Here's the drawing with two shaded views (mm, measured from the low corner). I have some questions. Round coordinates to 2 decimals unless told otherwise and drop trailing zeros. Loops run counter-clockwise (first coordinate to the right, second up) from the corner with the lowest first, then second, coordinate; pieces in that order, holes last.
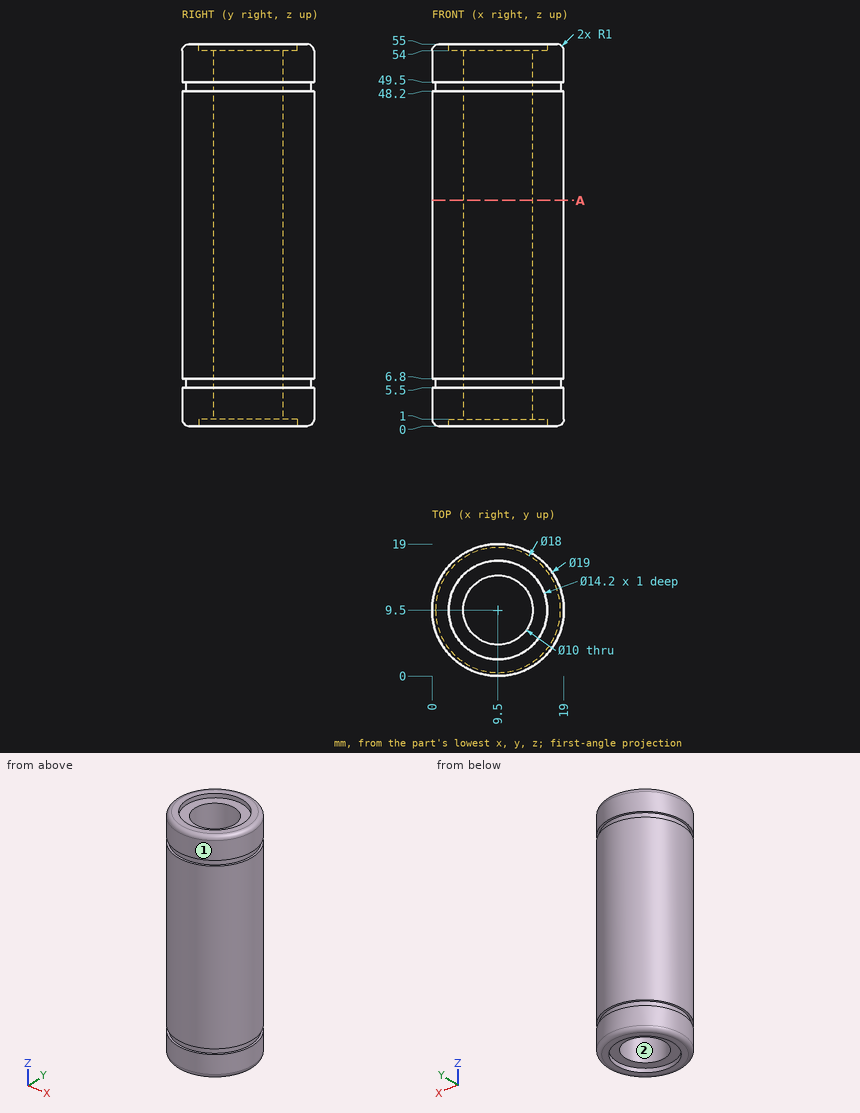
Item 1: If we section it at A-A, the plane z = 32.5: Please give me the cut outline in (x, y).
Results list:
outline: circle Ø19 at (9.5, 9.5); hole circle Ø10 at (9.5, 9.5)
Item 2: We'd pull the mould along X, two halves only. Please class the marked faces 1 and 2: released by +X, released by -X, zero draft, split by the parting line, or undercut.
Results list:
face 1: split by the parting line
face 2: undercut
Item 3: Will these pins go through, and if not, where does the flat tip stop? pin 1 (8 mm diameter, centred on x = 9.5, y = 9.5, fed in from +Z); pin 2 (1 mm diameter, centred on y = 7.5, z = 21.5, fed in from -X); pin 3 (1.5 mm diameter, centred on x = 11, z = 41.5, fed in from +Y); pin 4 (7 mm diameter, centred on x = 7, y = 10.5, fed in from +Z).
Results list:
pin 1: passes through
pin 2: stops at x = 0.12
pin 3: stops at y = 18.97
pin 4: stops at z = 54
Item 4: If I drill on line 1 along Y through (x, z) = (9.5, 16.5); line 2 along X through (y, z) = (10, 25); line 3 along Z through (x, y) = (15.5, 9), over which ranges is the centre line in solid material (lowest first)?
Results list:
line 1: y = 0 to 4.5, 14.5 to 19
line 2: x = 0.01 to 4.53, 14.47 to 18.99
line 3: z = 1 to 54
